```python
from build123d import *

# Parameters (mm, degrees)
BOSS_EXTRUDE1_DEPTH       = 6.35
M5_CLEARANCE_HOLE1_D      = 5.5
M5_CLEARANCE_HOLE1_DEPTH  = 12.7
M5_CLEARANCE_HOLE1_TIP    = 1.652366702
F_6_CLEARANCE_HOLE2_D     = 3.7973
F_6_CLEARANCE_HOLE2_DEPTH = 12.7
F_6_CLEARANCE_HOLE2_TIP   = 1.140824014
M5_CLEARANCE_HOLE2_D      = 5.5
M5_CLEARANCE_HOLE2_DEPTH  = 12.7
M5_CLEARANCE_HOLE2_TIP    = 1.652366702
FILLET1_R                 = 6.35
SKETCH8_R                 = 8
CUT_EXTRUDE1_DEPTH        = 6.35
SKETCH11_R                = 6.35
CUT_EXTRUDE2_DEPTH        = 6.35


with BuildPart() as part:
    # Sketch1 → Boss-Extrude1 (new body)
    with BuildSketch(Plane(origin=(0, 0, 0), x_dir=(1, 0, 0), z_dir=(0, 1, 0))):
        Polygon((-228.6, 12.7), (228.6, 12.7), (285.75, 12.7), (285.75, -59.055), (228.6, -59.055), (228.6, -12.7), (-228.6, -12.7), (-228.6, -38.1), (-279.4, -38.1), (-279.4, -12.7), (-292.1, -12.7), (-292.1, 12.7), (-279.4, 12.7), align=None)
    extrude(amount=BOSS_EXTRUDE1_DEPTH)

    # M5 Clearance Hole1
    with Locations(Plane(origin=(0, 6.35, 0), x_dir=(1, 0, 0), z_dir=(0, 1, 0))):
        with Locations((-270.167891819, -6.003039934), (-260.696960066, -28.867891819), (-237.832108181, -19.396960066), (-260.696960066, 3.467891819), (-247.303039934, 3.467891819), (-237.832108181, -6.003039934), (-270.167891819, -19.396960066), (-247.303039934, -28.867891819)):
            Hole(M5_CLEARANCE_HOLE1_D / 2, depth=M5_CLEARANCE_HOLE1_DEPTH)
            with Locations((0, 0, -(M5_CLEARANCE_HOLE1_DEPTH + M5_CLEARANCE_HOLE1_TIP / 2))):  # 118° drill point
                Cone(0, M5_CLEARANCE_HOLE1_D / 2, M5_CLEARANCE_HOLE1_TIP, mode=Mode.SUBTRACT)

    # #6 Clearance Hole2
    with Locations(Plane(origin=(0, 0, -12.7), x_dir=(-1, 0, 0), z_dir=(0, 0, -1))):
        with Locations((279.4, 3.175), (215.9, 3.175), (0, 3.175), (-215.9, 3.175), (-276.225, 3.175)):
            Hole(F_6_CLEARANCE_HOLE2_D / 2, depth=F_6_CLEARANCE_HOLE2_DEPTH)
            with Locations((0, 0, -(F_6_CLEARANCE_HOLE2_DEPTH + F_6_CLEARANCE_HOLE2_TIP / 2))):  # 118° drill point
                Cone(0, F_6_CLEARANCE_HOLE2_D / 2, F_6_CLEARANCE_HOLE2_TIP, mode=Mode.SUBTRACT)

    # M5 Clearance Hole2
    with Locations(Plane(origin=(0, 6.35, 0), x_dir=(1, 0, 0), z_dir=(0, 1, 0))):
        with Locations((218.475, -17.174999994), (218.475, -37.174999994), (244.475, -27.174999994), (256.475, -3.175), (256.475, -51.175), (236.475, -3.175), (236.475, -51.175), (270.475, -17.174999994), (270.475, -37.174999994)):
            Hole(M5_CLEARANCE_HOLE2_D / 2, depth=M5_CLEARANCE_HOLE2_DEPTH)
            with Locations((0, 0, -(M5_CLEARANCE_HOLE2_DEPTH + M5_CLEARANCE_HOLE2_TIP / 2))):  # 118° drill point
                Cone(0, M5_CLEARANCE_HOLE2_D / 2, M5_CLEARANCE_HOLE2_TIP, mode=Mode.SUBTRACT)

    # Fillet1
    fillet1_edges = [part.edges().sort_by_distance(p)[0] for p in [
        (285.75, 3.175, 59.055),
        (228.6, 3.175, 59.055),
        (228.6, 3.175, 12.7),
        (-228.6, 3.175, 12.7),
        (-228.6, 3.175, 38.1),
        (-279.4, 3.175, 38.1),
        (-279.4, 3.175, 12.7),
        (-292.1, 3.175, 12.7),
    ]]
    fillet(fillet1_edges, radius=FILLET1_R - 0.0001)  # a hair under: the kernel refuses the full size

    # Sketch8 → Cut-Extrude1 (cut)
    with BuildSketch(Plane(origin=(0, 6.35, 0), x_dir=(1, 0, 0), z_dir=(0, 1, 0))):
        with Locations(Location((-254, -12.7, 0), (0, 0, 270))):
            Circle(SKETCH8_R)
        with Locations(Location((244.475, -27.174999994, 0), (0, 0, 270))):
            Circle(SKETCH8_R)
    extrude(amount=-CUT_EXTRUDE1_DEPTH, mode=Mode.SUBTRACT)

    # Sketch11 → Cut-Extrude2 (cut)
    with BuildSketch(Plane(origin=(0, 6.35, 0), x_dir=(1, 0, 0), z_dir=(0, 1, 0))):
        with Locations(Location((-196.85, 0, 0), (0, 0, 270))):
            Circle(SKETCH11_R)
        with Locations(Location((-164.041666667, 0, 0), (0, 0, 270))):
            Circle(SKETCH11_R)
        with Locations(Location((-131.233333333, 0, 0), (0, 0, 270))):
            Circle(SKETCH11_R)
        with Locations(Location((-98.425, 0, 0), (0, 0, 270))):
            Circle(SKETCH11_R)
        with Locations(Location((-65.616666667, 0, 0), (0, 0, 270))):
            Circle(SKETCH11_R)
        with Locations(Location((-32.808333333, 0, 0), (0, 0, 270))):
            Circle(SKETCH11_R)
    cut_extrude2 = extrude(amount=-CUT_EXTRUDE2_DEPTH, mode=Mode.SUBTRACT)

    # Mirror1: Cut-Extrude2 across plane
    add(cut_extrude2.mirror(Plane(origin=(0, 0, 0), x_dir=(0, 0, 1), z_dir=(1, 0, 0))), mode=Mode.SUBTRACT)


solid = part.part
```
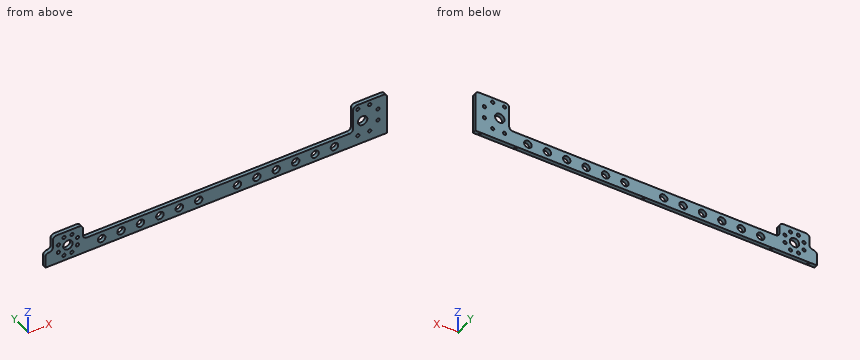
The model under review builds one solid part; all positions refer to its coordinate system, in mm. Round coordinates to 2 decimals unless told otherwise and drop trailing zeros. Order: outer loops, then holes, each group sorted by start corner. A loop starts at its lowest first (then second) coordinate and runs counter-clockwise, first axis right, second up. Notation, with made-up numbers: (-33, -16) -> (25, -16) arc R11 cw to (25, 1) -> close; hole circle Ø4 at (68.5, 7.25). An arc over 180 degrees is marked (long way). Use a Markdown table: item, result.
Q1. We need section A-A on x = 196.85. Write out the cut boundary in (y, z).
Values:
| item | result |
|---|---|
| outline | (0, -12.7) -> (6.35, -12.7) -> (6.35, -6.35) -> (0, -6.35) -> close; (0, 6.35) -> (6.35, 6.35) -> (6.35, 12.7) -> (0, 12.7) -> close |
Q2. For line 1 (X direction, y = 4.25, z = 20); line 2 (X direction, y = 1, z = 15.5); line 3 (Z direction, x = -48, y = 4.5), list the stretches that pass through material, from the lowest coordinate up.
Values:
| item | result |
|---|---|
| line 1 | x = -279.4 to -272.85, -267.48 to -257.27, -250.73 to -240.52, -235.15 to -228.6, 228.6 to 240.94, 248.01 to 285.75 |
| line 2 | x = -280.48 to -261.49, -246.51 to -227.52, 227.52 to 268.29, 272.66 to 285.75 |
| line 3 | z = -12.7 to 12.7 |
Q3. Clearance check with flat-ended pins moving along their axes: P1, Ø3.5, axis at x = 276.225, y = 3.175, coming from the -Z side; P2, Ø10, axis at x = 52.5, z = 22, coming from the +Y side. State where each tip first meets the part, or that it passes through.
Values:
| item | result |
|---|---|
| P1 | stops at z = 0.09 |
| P2 | passes through |
